Verification items for the finished model (mm, model axes). Round coordinates to 2 decimals unless told otherwise and drop trailing zeros. Write each loop counter-clockwise with the first axis right and the second up, starting at its lowest first coordinate (ties: lowest second). Pieces come first, ordered by that corner, then holes. Notation, with made-up numbers: M 43.5,-13.75 L 65.5,-13.75 A30 ccw 65.5,25.25 Z; hole C -27.5,67 d1. An arc over 180 degrees is marked long. One line per item, written item: value. Start each with the question number.
Item 1: Gauge pin test, flat ends, axial feed: pin 1 (5 mm diameter, centred on x = 25.5, y = -43, fed in from -Z); pin 2 (10 mm diameter, centred on y = 6.5, z = -9.5, fed in from -X). Record the tip position at first contact, or that the pin passes through.
Item 2: Section check A-A, the plane x = -2. Record the cut outline in (y, z).
Item 3: Thickness scan on probe 1 along Y at (x, z) = (-34, -15); probe 2 along Z at (x, y) = (-7, 71); probe 3 along X at (y, z) = (-71, -8). Record the ranges inside material, lowest first. Write a range as from..to.
Item 4: Draft check along X on faces 1 (the face through (-74, -73, -84.438)), 2 (the face through (44.712, -73.651, -44.067)). Enter one of: +X half, -X half, draft (parallel to the pull), parting line (faces both ways), or undercut.
Item 5: Section check B-B, the plane y = 3. Record the cut outline in (x, z), then the cut area to 3 significant figures.
Solid Edge part; units mm, degrees
sketch "Sketch1" plane through (0, 0, 0) normal (0, 0, 1) x (1, 0, 0)
  line L0 (32.5, 80) -> (-32.5, 80)
  line L1 (-32.5, 80) -> (-32.5, -80)
  line L2 (-32.5, -80) -> (32.5, -80)
  line L3 (32.5, -80) -> (32.5, 80)
  dimension "D1" = 32.5
  dimension "D2" = 32.5
extrude "Protrusion1" add sketch "Sketch1" along normal blind 1
sketch "Sketch2" plane through (5.2285, 0, 16.7452) normal (0.5, 0, 0.8660254) x (0, 1, 0)
  circle A0 centre (-73, 17.8013) radius 5
extrude "ProtrusioneEstrusa_4" add sketch "Sketch2" against normal blind 130
mirror "Mirror1" about plane through (0, 0, 0) normal (1, 0, 0) of "ProtrusioneEstrusa_4"
mirror "Mirror2" about plane through (0, 0, 0) normal (0, -1, 0) of "Mirror1", "ProtrusioneEstrusa_4"
sketch "Sketch3" plane through (0, -80, 1.5) normal (0, -1, 0) x (1, 0, 0)
  line L0 (32.5, 26.6458) -> (-32.5, 26.6458)
  line L1 (-32.5, 26.6458) -> (-32.5, -0.5)
  line L2 (-32.5, -0.5) -> (32.5, -0.5)
  line L3 (32.5, -0.5) -> (32.5, 26.6458)
extrude "Cutout1" cut sketch "Sketch3" against normal through all
sketch "Sketch4" plane through (0, -80, 1.5) normal (0, -1, 0) x (1, 0, 0)
  line L0 (79.5179, -85.9375) -> (-79.5179, -85.9375)
  line L1 (-79.5179, -85.9375) -> (-79.5179, -90.9375)
  line L2 (-79.5179, -90.9375) -> (79.5179, -90.9375)
  line L3 (79.5179, -90.9375) -> (79.5179, -85.9375)
extrude "Cutout2" cut sketch "Sketch4" against normal through all
properties material "Fe 360 B UNI 7070"
Response values:
1. pin 1: stops at z = 0
1. pin 2: passes through
2. outline: M -80,0 L 80,0 L 80,1 L -80,1 Z
3. probe 1: y = -77.99..-68.01, 68.01..77.99
3. probe 2: z = 0..1
3. probe 3: x = -34.9..-24.32, 24.32..34.9
4. face 1: draft
4. face 2: undercut
5. outline: M -32.5,0 L 32.5,0 L 32.5,1 L -32.5,1 Z
5. area: 65.0 mm2
